from build123d import *

# Parameters (mm, degrees)
BOSS_EXTRUDE1_DEPTH = 3


with BuildPart() as part:
    # Sketch2 → Boss-Extrude1 (new body)
    with BuildSketch(Plane(origin=(0, 0, 0), x_dir=(1, 0, 0), z_dir=(0, 1, 0))):
        with BuildLine():
            Line((0, 0), (0, 12.875))
            Line((0, 12.875), (-3, 12.875))
            Line((-3, 12.875), (-3, 25.575))
            Line((-3, 25.575), (0, 25.575))
            Line((0, 25.575), (0, 41.45))
            ThreePointArc((0, 41.45), (13.737406392, 22.614642557), (19.4, 0))
            Line((19.4, 0), (12.266745701, 0))
            Line((12.266745701, 0), (12.266745701, -3))
            Line((12.266745701, -3), (7.186745701, -3))
            Line((7.186745701, -3), (7.186745701, 0))
            Line((7.186745701, 0), (0, 0))
        make_face()
    extrude(amount=BOSS_EXTRUDE1_DEPTH)


solid = part.part
The model under review builds one solid part; all positions refer to its coordinate system, in mm. A direction names the side the tool comes from. Give positions to 0.01 mm unless a question says otherwise; leave off trailing zeros. Loops run counter-clockwise (first coordinate to the right, second up) from the corner with the lowest first, then second, coordinate; pieces in that order, holes last. Notation, with made-up numbers: (61, 21) -> (105, 21) arc R27 ccw to (105, 43) -> close; hole circle Ø2 at (-9, -30.75). An arc over 180 degrees is marked (long way). Put each result on its own line as item: value. Start each with the question number.
1. Clearance check with flat-ended pins moving along their axes: P1, Ø1, axis at x = 6.5, y = 0.5, coming from the +Z side; P2, Ø1.5, axis at x = 1, z = -26, coming from the -Y side; P3, Ø1.5, axis at x = -1.5, y = 1.5, coming from the +Z side (3 decimals); P4, Ø1.5, axis at y = 2, z = 2, coming from the +X side. State where each tip first meets the part, or that it passes through.
2. We need section A-A on y = 1.7. State the section outline as (x, z) points (3 decimals).
3. Wall thickness on probe 1 along X at (y, z) = (2.5, 1); probe 2 along X at (y, z) = (1.7, -12); probe 3 along Z at (x, y) = (3.5, 1.6): over which ranges is each line inside the solid? List them lowest first.
4. We need section C-C on z = -38. State the section outline as (x, y) points, then the cut area to 3 significant figures.
5. We need section B-B on x = -0.5. State the section outline as (y, z) points (3 decimals).
6. For faces 1 (the face through (4, 1, 0)), 2 (the face through (0, 1, -33)), 3 (the face through (12.267, 1, 1)), 4 (the face through (-3, 1, -19)), 5 (the face through (13.6, 1.48, -22.91)), list the 3-axis set-ups (+Z, -Z, +X, -X, +Y, -Y) from which the entire face can be reached by the end or side of a thin tool; tool diameter is ignored.
Determined:
1. P1: z = 0
1. P2: y = 0
1. P3: z = -12.875
1. P4: x = 12.27
2. outline: (-3, -25.575) -> (0, -25.575) -> (0, -41.45) arc R60.96 ccw to (19.4, 0) -> (12.267, 0) -> (12.267, 3) -> (7.187, 3) -> (7.187, 0) -> (0, 0) -> (0, -12.875) -> (-3, -12.875) -> close
3. probe 1: 7.19 to 12.27
3. probe 2: 0 to 17.55
3. probe 3: -37.92 to 0
4. outline: (0, 0) -> (3.43, 0) -> (3.43, 3) -> (0, 3) -> close
4. area: 10.3 mm^2
5. outline: (0, -25.575) -> (3, -25.575) -> (3, -12.875) -> (0, -12.875) -> close
6. face 1: +Z, -X, +Y, -Y
6. face 2: -Z, -X, +Y, -Y
6. face 3: +Z, +X, +Y, -Y
6. face 4: +Z, -Z, -X, +Y, -Y
6. face 5: -Z, +X, +Y, -Y
